Verification items for the finished model (mm, model axes). Face numbers are marked on the shaded views. A direction names the side the tool comes from. Give positions to 0.01 mm unless a question says otherwise; leave off trailing zeros. Loops run counter-clockwise (first coordinate to the right, second up) from the corner with the lowest first, then second, coordinate; pieces in that order, holes last. Notation, with made-up numbers: (-10, 84) - (17, 84) arc R7 cw to (17, 93) - close; hole circle Ø5 at (18.25, -39.75). An arc over 180 degrees is marked (long way). Use one line per item in the form item = value.
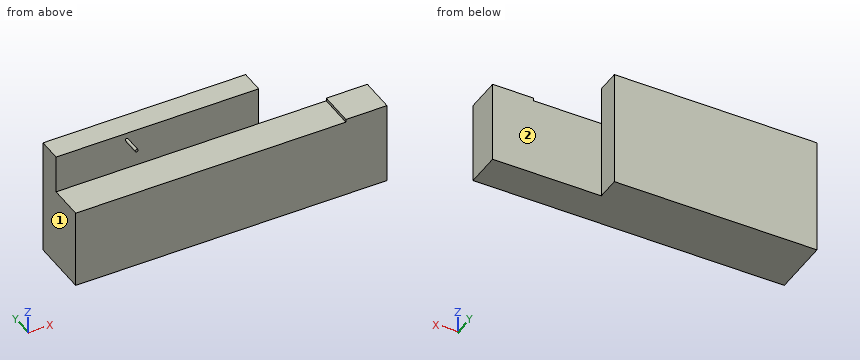
```python
from build123d import *

# Parameters (mm, degrees)
F1_DEPTH = 673.1
F2_W     = 234.95
F2_H     = 50.8
F3_DEPTH = 254.001
F4_W     = 88.9
F4_H     = 76.2
F5_DEPTH = 6.35
F6_R     = 3.175
F7_DEPTH = 38.52672


with BuildPart() as f1:
    # F0 (on Right) → F1 (new body)
    with BuildSketch(Plane.YZ):
        Polygon((-63.5, 44.45), (-63.5, -127), (63.5, -127), (63.5, 127), (12.7, 127), (12.7, 44.45), align=None)
    extrude(amount=F1_DEPTH)

    # F2 (on face) → F3 (cut, through all)
    with BuildSketch(Plane.XY.offset(127)):
        with Locations((555.625, 38.1)):
            Rectangle(F2_W, F2_H)
    extrude(amount=-F3_DEPTH, mode=Mode.SUBTRACT)

    # F4 (on face) → F5 (join)
    with BuildSketch(Plane.XY.offset(44.45)):
        with Locations((628.65, -25.4)):
            Rectangle(F4_W, F4_H)
    extrude(amount=F5_DEPTH)

    # F6 (on face) → F7 (join)
    with BuildSketch(Plane.XZ.offset(-12.7)):
        with Locations((152.781, 111.4806)):
            Circle(F6_R)
    extrude(amount=F7_DEPTH)


solid = f1.part
```
1. Section check D-D, the plane y = 50. Record the cut outline in (x, z).
Result set:
outline = (0, -127) - (438.15, -127) - (438.15, 127) - (0, 127) - close
2. Tool access check on the marked faces 1 and 2. Record the directions out of +Z, -Z, +X, -X, +Y, -Y that give a thin tool (end or side, any length) a straight path to the whole face; none if there is none.
Result set:
face_1 = +Z, -Z, -X, +Y, -Y
face_2 = +Z, -Z, +X, +Y
3. Section check B-B, the plane z = -54. Record the cut outline in (x, y).
Result set:
outline = (0, -63.5) - (673.1, -63.5) - (673.1, 12.7) - (438.15, 12.7) - (438.15, 63.5) - (0, 63.5) - close
4. Section check C-C, the plane x = 411. Record the cut outline in (y, z).
Result set:
outline = (-63.5, -127) - (63.5, -127) - (63.5, 127) - (12.7, 127) - (12.7, 44.45) - (-63.5, 44.45) - close
5. Scan lines: probe 1 along Y at (x, z) = (504, -84); probe 2 along Z at (x, y) = (196, -49.5); probe 3 along Y at (x, z) = (103, 78). Record each from-to range of solid material in increasing order.
Result set:
probe_1 = -63.5 to 12.7
probe_2 = -127 to 44.45
probe_3 = 12.7 to 63.5
6. Section check A-A, the plane y = -17. Record the cut outline in (x, z) (3 decimals), then the cut area to 3 significant figures.
Result set:
outline = (0, -127) - (673.1, -127) - (673.1, 50.8) - (584.2, 50.8) - (584.2, 44.45) - (0, 44.45) - close; circle Ø6.35 at (152.781, 111.481)
area = 116,000 mm²
7. Depth check by flat-ended pin: pin 1 Ø23 at (x, y) = (289, -40.5) entering from +Z; pin 2 Ø3 at (x, z) = (153.5, 111.5) entering from -Y; pin 3 Ø3 at (y, z) = (-20.5, 46.5) entering from -X. Enter the tip coordinate at first touch or a pass-through.
Result set:
pin_1 = 44.45
pin_2 = -25.83
pin_3 = 584.2
